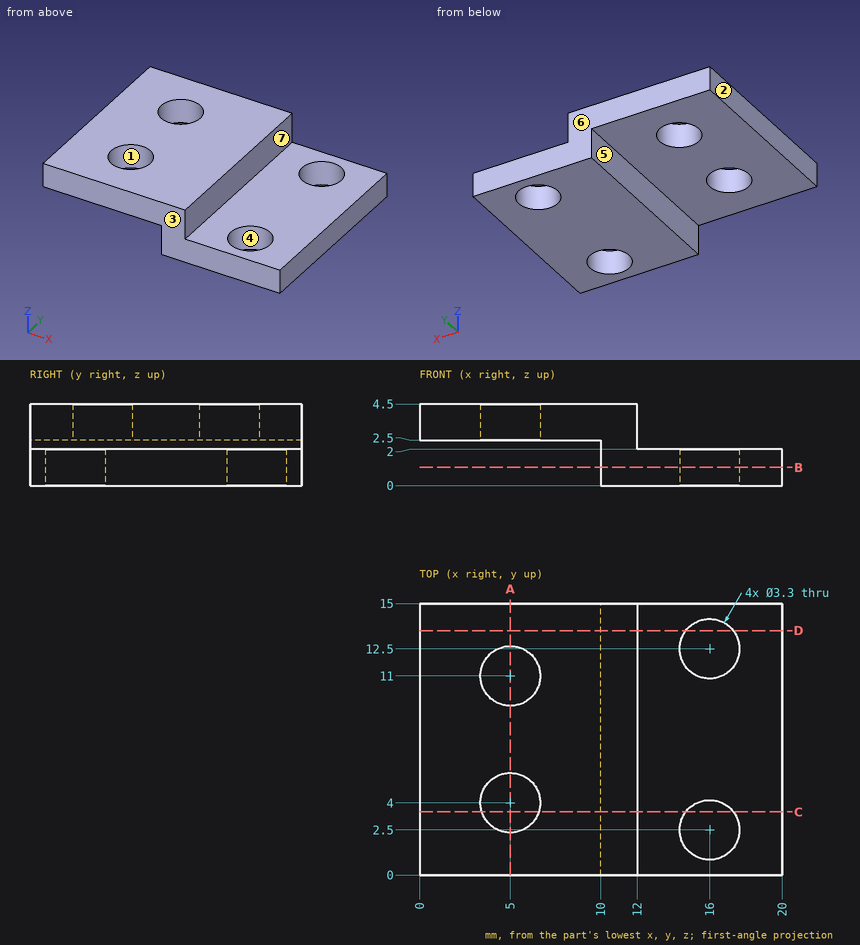
Drawing for the job (mm, zero at the part's lowest x, y, z). A direction names the side the tool comes from. Give positions to 0.01 mm unless a question says otherwise; leave off trailing zeros. Order: outer loops, then holes, each group sorted by start corner. A loop starts at its lowest first (then second) coordinate and runs counter-clockwise, first axis right, second up. Notation, with made-up numbers: M 32.25,37.25 L 63.25,37.25 A25 cw 63.25,61.25 Z; hole C 69,-19.75 d10. An arc over 180 degrees is marked long. Use a Markdown table: item, result. Add a question column.
(1) 3-axis set-ups, long thin cutter, end or side, ignore diameter. For the marked faces 5, 6 and 7: which of +Z, -Z, +X, -X, +Y, -Y reach the whole face in a straight line?
(2) Saw through at A-A, the plane x = 5. Give the cut face in (y, z).
(3) Saw through at D-D, the plane y = 13.5. Give the cut face in (x, z), and give its area (3 significant figures).
(4) Saw through at C-C, the plane y = 3.5. Give the cut face in (x, z).
(5) Mould opens along Y. For the marked faces 1, 2, 3 and 4 say: +Y half, -Y half, draft (parallel to the pull), parting line (faces both ways), or undercut.
(6) Probe line 1 along Y through (x, z) = (5, 3.6); line 2 along Y through (x, z) = (16, 1.6); line 3 along Z through (x, y) = (5, 8). List the from-to ranges inside material, lowest first. Write a range as [from, to].
(7) Drop flat-ended pins along their axis: P1, Ø3, axis at x = 16, y = 12.5, coming from the +Z side; P2, Ø1.5, axis at y = 8, z = 3, coming from the +X side; P3, Ø8, axis at x = 3, y = 6, coming from the -Z side; P4, Ø4, axis at x = 17.5, y = 10, coming from the +Z side. Give the stop position or say it passes through.
(8) Saw through at B-B, the plane z = 1. Give the cut face in (x, y).
Answer key:
| question | item | result |
|---|---|---|
| 1 | face 5 | -Z, -X, +Y, -Y |
| 1 | face 6 | +Z, -Z, +X, -X, +Y |
| 1 | face 7 | +Z, +X, +Y, -Y |
| 2 | outline | M 0,2.5 L 2.35,2.5 L 2.35,4.5 L 0,4.5 Z; M 5.65,2.5 L 9.35,2.5 L 9.35,4.5 L 5.65,4.5 Z; M 12.65,2.5 L 15,2.5 L 15,4.5 L 12.65,4.5 Z |
| 3 | outline | M 0,2.5 L 10,2.5 L 10,0 L 14.69,0 L 14.69,2 L 12,2 L 12,4.5 L 0,4.5 Z; M 17.31,0 L 20,0 L 20,2 L 17.31,2 Z |
| 3 | area | 39.8 mm^2 |
| 4 | outline | M 0,2.5 L 3.43,2.5 L 3.43,4.5 L 0,4.5 Z; M 6.57,2.5 L 10,2.5 L 10,0 L 14.69,0 L 14.69,2 L 12,2 L 12,4.5 L 6.57,4.5 Z; M 17.31,0 L 20,0 L 20,2 L 17.31,2 Z |
| 5 | face 1 | undercut |
| 5 | face 2 | draft |
| 5 | face 3 | -Y half |
| 5 | face 4 | undercut |
| 6 | line 1 | [0, 2.35], [5.65, 9.35], [12.65, 15] |
| 6 | line 2 | [0, 0.85], [4.15, 10.85], [14.15, 15] |
| 6 | line 3 | [2.5, 4.5] |
| 7 | P1 | through |
| 7 | P2 | x = 12 |
| 7 | P3 | z = 2.5 |
| 7 | P4 | z = 2 |
| 8 | outline | M 10,0 L 20,0 L 20,15 L 10,15 Z; hole C 16,2.5 d3.3; hole C 16,12.5 d3.3 |
